The model under review builds one solid part; all positions refer to its coordinate system, in mm. Round coordinates to 2 decimals unless told otherwise and drop trailing zeros. Loops run counter-clockwise (first coordinate to the right, second up) from the corner with the lowest first, then second, coordinate; pieces in that order, holes last. Notation, with made-up numbers: M -7,86.5 L 1,86.5 A26 cw 1,124.5 Z; hole C 49.25,52 d1. An arc over 180 degrees is marked long. Answer in a Markdown table with one row per item. Add a question column.
from build123d import *

# Parameters (mm, degrees)
CROQUIS1_R              = 100
SALIENTE_EXTRUIR1_DEPTH = 3
CROQUIS3_R              = 110
CORTAR_EXTRUIR1_DEPTH   = 3
REDONDEO1_R             = 10


with BuildPart() as part:
    # Croquis1 → Saliente-Extruir1 (new body)
    with BuildSketch(Plane.XY):
        Circle(CROQUIS1_R)
    extrude(amount=SALIENTE_EXTRUIR1_DEPTH)

    # Croquis3 → Cortar-Extruir1 (cut)
    with BuildSketch(Plane.XY.offset(3)):
        with Locations((190, 0)):
            Circle(CROQUIS3_R)
    extrude(amount=-CORTAR_EXTRUIR1_DEPTH, mode=Mode.SUBTRACT)

    # Redondeo1
    redondeo1_edges = [part.edges().sort_by_distance(p)[0] for p in [
        (89.473684211, -44.659375654, 1.5),
        (89.473684211, 44.659375654, 1.5),
    ]]
    fillet(redondeo1_edges, radius=REDONDEO1_R)


solid = part.part
1. Take a section at A-A, the plane y = 0. State the section outline as (x, z) points, and give its area (3 significant figures).
2. For pin 1 Ø1.5 at (x, z) = (-45, 2) entering from -Y; pin 2 Ø1.5 at (y, z) = (11, 2) entering from +X, all flat-tipped, find the tip position at first contact; note any pin that passes through.
3. Take a section at B-B, the plane x = -47.5. State the section outline as (y, z) points, and give its area (3 significant figures).
4. Mouldability with a two-part tool opening along Y and no side actions: class faces 1 (the flat face through (-7, 1, 0)), 2 (the cylindrical face through (80, 0.6, 1.5)), 3 (the cylindrical face through (-99.932, 3.679, 1.479)) as released by +Y, released by -Y, zero draft, split by the parting line, or undercut.
5. To check wall thickness, follow probe 1 along X at (y, z) = (2.5, 1.15); probe 2 along X at (y, z) = (25, 1.6); probe 3 along Y at (x, z) = (-6, 1.45). State the ranges of each line that lie inside material, in increasing order.
Check sheet entries:
| question | item | result |
|---|---|---|
| 1 | outline | M -100,0 L 80,0 L 80,3 L -100,3 Z |
| 1 | area | 540 mm^2 |
| 2 | pin 1 | stops at y = -89.68 |
| 2 | pin 2 | stops at x = 80.63 |
| 3 | outline | M -88,0 L 88,0 L 88,3 L -88,3 Z |
| 3 | area | 528 mm^2 |
| 4 | face 1 | zero draft |
| 4 | face 2 | undercut |
| 4 | face 3 | split by the parting line |
| 5 | probe 1 | x = -99.97 to 80.03 |
| 5 | probe 2 | x = -96.82 to 82.88 |
| 5 | probe 3 | y = -99.82 to 99.82 |
